Source: CAD feature listing. Evaluate the final solid. Frame: model axes, mm. Face numbers are marked on the shaded views. A direction names the side the tool comes from. Give positions to 0.01 mm unless a question says otherwise; leave off trailing zeros. Write each loop counter-clockwise with the first axis right and the second up, starting at its lowest first coordinate (ties: lowest second). Pieces come first, ordered by that corner, then holes. Notation, with made-up numbers: M 16,34 L 72,34 A25 ccw 72,46 Z; hole C -38,38.5 d10. An arc over 180 degrees is marked long. Use CSV: the item, a comma, the result in double quotes. Start each with the question number.
from build123d import *

# Parameters (mm, degrees)
F0_W     = 150
F0_H     = 71
F1_DEPTH = 2
F2_W     = 150
F2_H     = 71
F2_W_2   = 144
F2_H_2   = 65
F3_DEPTH = 40
F4_W     = 1
F4_H     = 65
F5_DEPTH = 40
F6_W     = 1
F6_H     = 65
F7_DEPTH = 40


with BuildPart() as f1:
    # F0 (on Top) → F1 (new body)
    with BuildSketch(Plane.XY):
        with Locations((75, 35.5)):
            Rectangle(F0_W, F0_H)
    extrude(amount=F1_DEPTH)

    # F2 (on face) → F3 (join)
    with BuildSketch(Plane.XY.offset(2)):
        with Locations((75, 35.5)):
            Rectangle(F2_W, F2_H)
        with Locations((75, 35.5)):
            Rectangle(F2_W_2, F2_H_2, mode=Mode.SUBTRACT)
    extrude(amount=F3_DEPTH)

    # F4 (on face) → F5 (join)
    with BuildSketch(Plane.XY.offset(2)):
        with Locations((21.6, 35.5)):
            Rectangle(F4_W, F4_H)
    extrude(amount=F5_DEPTH)

    # F6 (on face) → F7 (join)
    with BuildSketch(Plane.XY.offset(2)):
        with Locations((40.7, 35.5)):
            Rectangle(F6_W, F6_H)
        with Locations((58.8, 35.5)):
            Rectangle(F6_W, F6_H)
        with Locations((76.9, 35.5)):
            Rectangle(F6_W, F6_H)
        with Locations((95, 35.5)):
            Rectangle(F6_W, F6_H)
        with Locations((113.1, 35.5)):
            Rectangle(F6_W, F6_H)
        with Locations((131.2, 35.5)):
            Rectangle(F6_W, F6_H)
    extrude(amount=F7_DEPTH)


solid = f1.part
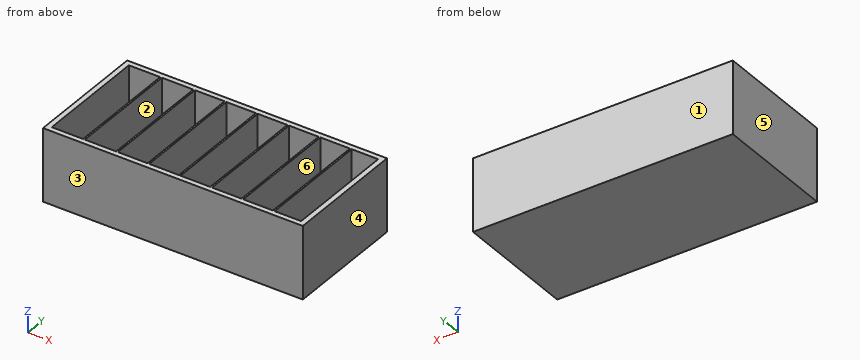
1. First-contact query: pin 1 (8 mm diameter, centred on x = 67.5, y = 62, fed in from -Z); pin 2 (8.5 mm diameter, centred on x = 85, y = 36.5, fed in from +Z). Flat tips, straight axial feed; report the tip coordinate or a pass-through.
2. Section A-A on x = 68. Return loops of the section in (y, z), then the cut area to 3 significant figures.
3. Line query: probe 1 along Y at (x, z) = (37.5, 17.5); probe 2 along Z at (x, y) = (111.5, 10). Output: solid intervals per line, ascending.
4. Section B-B on z = 27.5. Give the number of separate pieces and of enclosed holes in the cut face, then the cut area to 4 significant figures.
5. Pull-direction query (X, two-part tool) for the marked faces 3, 4, 5 and 6; classes: released by +X, released by -X, zero draft, split by the parting line, or undercut.
6. Access query for the marked faces 1 and 2. Directions: +Z, -Z, +X, -X, +Y, -Y. A direction counts if a zero-diameter tool reaches every point of the face in a straight line with its end or side. Return the directions, or none.
Resolved:
1,pin 1,"stops at z = 0"
1,pin 2,"stops at z = 2"
2,outline,"M 0,0 L 71,0 L 71,42 L 68,42 L 68,2 L 3,2 L 3,42 L 0,42 Z"
2,area,"382 mm2"
3,probe 1,"y = 0 to 3, 68 to 71"
3,probe 2,"z = 0 to 2"
4,separate pieces,"1"
4,enclosed holes,"8"
4,area,"1,745 mm2"
5,face 3,"zero draft"
5,face 4,"released by +X"
5,face 5,"released by -X"
5,face 6,"undercut"
6,face 1,"+Z, -Z, +X, -X, +Y"
6,face 2,"+Z"
